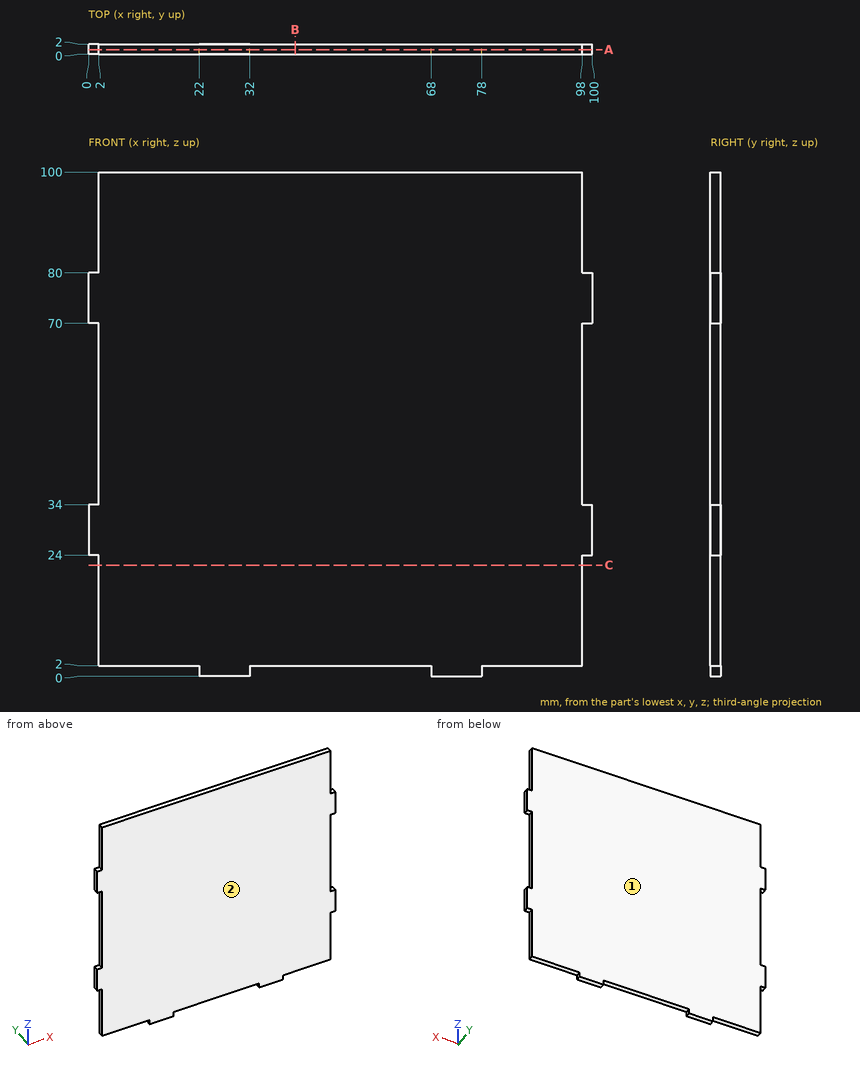
Design review of the part shown in the three views and the two pictorial views. Dimensions are in mm from the part's minimum x, y and z. Coordinates: 2 decimals unless noted, no trailing zeros. Loops run counter-clockwise (first coordinate to the right, second up) from the corner with the lowest first, then second, coordinate; pieces in that order, holes last. Notation, with made-up numbers: (27.25, 53) - (53.25, 53) arc R16 ccw to (53.25, 82) - close; hole circle Ø4 at (14.25, 22). An arc over 180 degrees is marked (long way). Use a Markdown table: item, result. Add a question column.
Item 1: For line 1 (X direction, y = 1.05, z = 55); line 2 (Z direction, x = 53.5, y = 1.65), list the stretches that pass through material, from the lowest coordinate up.
Item 2: Mouldability with a two-part tool opening along Y and no side actions: class the marked faces 1 and 2 as pulls with the +Y half, pulls with the -Y half, needs draft (parallel to the pull), parting line crosses it, or undercut.
Item 3: Insertion check: pin 1 Ø0.6 at (x, y) = (99, 1) entering from +Z; pin 2 Ø1 at (y, z) = (1, 44) entering from +X; pin 3 Ø4 at (x, z) = (47, 14) entering from -Y; pin 4 Ø1 at (x, y) = (99, 1) entering from -Z. Each pin has a flat end and moves straight along its axis. Give the tip position at first contact, or say it passes through.
Item 4: We need section A-A (y = 0.9). Give the boundary of the cut face in (x, z).
Item 5: We need section C-C (z = 22). Give the boundary of the cut face in (x, y), and give its area (3 significant figures).
Item 6: We need section B-B (x = 41). Give the boundary of the cut face in (y, z).
Results list:
| question | item | result |
|---|---|---|
| 1 | line 1 | x = 2 to 98 |
| 1 | line 2 | z = 2 to 100 |
| 2 | face 1 | pulls with the +Y half |
| 2 | face 2 | pulls with the -Y half |
| 3 | pin 1 | stops at z = 80 |
| 3 | pin 2 | stops at x = 98 |
| 3 | pin 3 | stops at y = 0 |
| 3 | pin 4 | stops at z = 24 |
| 4 | outline | (0, 24) - (2, 24) - (2, 2) - (22, 2) - (22, 0) - (32, 0) - (32, 2) - (68, 2) - (68, 0) - (78, 0) - (78, 2) - (98, 2) - (98, 24) - (100, 24) - (100, 34) - (98, 34) - (98, 70) - (100, 70) - (100, 80) - (98, 80) - (98, 100) - (2, 100) - (2, 80) - (0, 80) - (0, 70) - (2, 70) - (2, 34) - (0, 34) - close |
| 5 | outline | (2, 0) - (98, 0) - (98, 2) - (2, 2) - close |
| 5 | area | 192 mm^2 |
| 6 | outline | (0, 2) - (2, 2) - (2, 100) - (0, 100) - close |
